from build123d import *

# Parameters (mm, degrees)
SKETCH1_W           = 25.4
SKETCH1_H           = 25.4
BOSS_EXTRUDE1_DEPTH = 3
SKETCH2_R           = 1.778
SKETCH2_W           = 3
SKETCH2_H           = 6.35
SKETCH2_W_2         = 5.08
SKETCH2_H_2         = 3
CUT_EXTRUDE1_DEPTH  = 19.209338264


with BuildPart() as part:
    # Sketch1 → Boss-Extrude1 (new body)
    with BuildSketch(Plane.XY):
        Rectangle(SKETCH1_W, SKETCH1_H)
    extrude(amount=BOSS_EXTRUDE1_DEPTH)

    # Sketch2 → Cut-Extrude1 (cut, through all)
    with BuildSketch(Plane.XY.offset(3)):
        with Locations((-11.2, 0)):
            Circle(SKETCH2_R)
        with Locations((11.2, 0)):
            Circle(SKETCH2_R)
        with Locations((11.2, 9.525)):
            Rectangle(SKETCH2_W, SKETCH2_H)
        with Locations((11.2, -9.525)):
            Rectangle(SKETCH2_W, SKETCH2_H)
        with Locations((-11.2, 9.525)):
            Rectangle(SKETCH2_W, SKETCH2_H)
        with Locations((-11.2, -9.525)):
            Rectangle(SKETCH2_W, SKETCH2_H)
        with Locations((0, -10.16)):
            Rectangle(SKETCH2_W_2, SKETCH2_H_2)
    extrude(amount=-CUT_EXTRUDE1_DEPTH, mode=Mode.SUBTRACT)


solid = part.part
Work out the finished part from the listing and answer in its coordinate system (mm). A direction names the side the tool comes from. Round coordinates to 2 decimals unless told otherwise and drop trailing zeros. Write each loop counter-clockwise with the first axis right and the second up, starting at its lowest first coordinate (ties: lowest second). Pieces come first, ordered by that corner, then holes.
1) A cutting plane is placed at B-B (z = 1.6). Give the vertices of the cut face in (x, y), plus the area to 3 significant figures.
2) Given pin 1 Ø0.9 at (y, z) = (-10.5, 1) entering from -X; pin 2 Ø0.9 at (y, z) = (9, 1.5) entering from +X; pin 3 Ø0.9 at (x, z) = (-11, 2) entering from -Y, each flat-ended and moving along its own axis, determine where each tip first touches the part or whether it passes through.
3) The mould has two halves that part along X. Classify faces 5 (the cylindrical face through (9.423, 0.064, 1.521)), 6 (the flat face through (9.7, -10, 2)), 7 (the flat face through (-11, -6.35, 2)), 8 (the flat face through (2.54, -10, 2)): pulls with the +X half, pulls with the -X half, needs draft (parallel to the pull), parting line crosses it, or undercut.
4) A cutting plane is placed at A-A (y = -10.25). Give the vertices of the cut face in (x, z), plus the area to 3 significant figures.
5) A tool of negligible diameter and unlimited length cuts with its end or side. For faces 1 (the flat face through (11, -6.35, 2)), 2 (the flat face through (-9.7, 9, 2)), 3 (the flat face through (0, -11.66, 2)), 4 (the flat face through (11, 6.35, 2)), from which of +Z, -Z, +X, -X, +Y, -Y can it reach the whole face along a straight path? Write none if from no direction.
6) A cutting plane is placed at D-D (y = 0). Give the vertices of the cut face in (x, z), plus the area to 3 significant figures.
7) Straight lines are drawn through the part: line 1 (Y direction, x = -11.2, z = 2.2); line 2 (X direction, y = -10, z = 2.8); line 3 (Y direction, x = -2, z = 1.95). For each, find the intervals that lie inside material, in ascending order.
8) A cutting plane is placed at C-C (x = 2.25). Give the vertices of the cut face in (y, z), plus the area to 3 significant figures.
Completed:
1. outline: (-12.7, -6.35) - (-9.7, -6.35) - (-9.7, -12.7) - (9.7, -12.7) - (9.7, -6.35) - (12.7, -6.35) - (12.7, -0.95) arc R1.78 cw (long way) to (12.7, 0.95) - (12.7, 6.35) - (9.7, 6.35) - (9.7, 12.7) - (-9.7, 12.7) - (-9.7, 6.35) - (-12.7, 6.35) - (-12.7, 0.95) arc R1.78 cw (long way) to (-12.7, -0.95) - close; hole (-2.54, -11.66) - (2.54, -11.66) - (2.54, -8.66) - (-2.54, -8.66) - close
1. area: 535 mm2
2. pin 1: stops at x = -9.7
2. pin 2: stops at x = 9.7
2. pin 3: stops at y = -6.35
3. face 5: undercut
3. face 6: pulls with the +X half
3. face 7: needs draft
3. face 8: undercut
4. outline: (-9.7, 0) - (-2.54, 0) - (-2.54, 3) - (-9.7, 3) - close; (2.54, 0) - (9.7, 0) - (9.7, 3) - (2.54, 3) - close
4. area: 43.0 mm2
5. face 1: +Z, -Z, +X, -Y
5. face 2: +Z, -Z, -X, +Y
5. face 3: +Z, -Z
5. face 4: +Z, -Z, +X, +Y
6. outline: (-9.42, 0) - (9.42, 0) - (9.42, 3) - (-9.42, 3) - close
6. area: 56.5 mm2
7. line 1: y = -6.35 to -1.78, 1.78 to 6.35
7. line 2: x = -9.7 to -2.54, 2.54 to 9.7
7. line 3: y = -12.7 to -11.66, -8.66 to 12.7
8. outline: (-12.7, 0) - (-11.66, 0) - (-11.66, 3) - (-12.7, 3) - close; (-8.66, 0) - (12.7, 0) - (12.7, 3) - (-8.66, 3) - close
8. area: 67.2 mm2
